from build123d import *

# Parameters (mm, degrees)
ESQUISSE1_R                  = 25
BOSS_EXTRU_1_DEPTH           = 14
ENL_V_START                  = 26
ESQUISSE2_W                  = 9
ESQUISSE2_H                  = 9
ENL_V_MAT_EXTRU_1_DEPTH      = 16
R_P_TITION_CIRCULAIRE1_COUNT = 3
ESQUISSE9_R                  = 11.25
ENL_V_MAT_EXTRU_2_DEPTH      = 16
BOSS_EXTRU_3_START           = -14
BOSS_EXTRU_3_DEPTH           = 20


with BuildPart() as part:
    # Esquisse1 → Boss.-Extru.1 (new body)
    with BuildSketch(Plane.XY):
        Circle(ESQUISSE1_R)
    extrude(amount=BOSS_EXTRU_1_DEPTH)

    # Esquisse2 → Enlèv. mat.-Extru.1 (cut)
    with BuildSketch(Plane(origin=(0, 0, 0), x_dir=(0, 0, -1), z_dir=(1, 0, 0)).offset(ENL_V_START)):
        with Locations((-7, 0)):
            Rectangle(ESQUISSE2_W, ESQUISSE2_H)
    enl_v_mat_extru_1 = extrude(amount=-ENL_V_MAT_EXTRU_1_DEPTH, mode=Mode.SUBTRACT)

    # Répétition circulaire1: Enlèv. mat.-Extru.1 ×3 about axis
    r_p_tition_circulaire1_axis = Axis((0, 0, 0), (0, 0, 1))
    for i in range(1, R_P_TITION_CIRCULAIRE1_COUNT):
        add(enl_v_mat_extru_1.rotate(r_p_tition_circulaire1_axis, i * 360 / R_P_TITION_CIRCULAIRE1_COUNT), mode=Mode.SUBTRACT)

    # Esquisse9 → Enlèv. mat.-Extru.2 (cut)
    with BuildSketch(Plane(origin=(0, 0, 0), x_dir=(-1, 0, 0), z_dir=(0, 0, -1))):
        Circle(ESQUISSE9_R)
    extrude(amount=-ENL_V_MAT_EXTRU_2_DEPTH, mode=Mode.SUBTRACT)

    # Esquisse10 → Boss.-Extru.3 (add)
    with BuildSketch(Plane(origin=(0, 0, 0), x_dir=(-1, 0, 0), z_dir=(0, 0, -1)).offset(BOSS_EXTRU_3_START)):
        Polygon((-15.932437345, 19.265446796), (-21.202216656, 13.246358325), (-17.440286362, 9.952746256), (-12.170507051, 15.971834726), align=None)
    extrude(amount=-BOSS_EXTRU_3_DEPTH)


solid = part.part
Build history of the part. All positions in model axes, mm. A direction names the side the tool comes from. Round coordinates to 2 decimals unless told otherwise and drop trailing zeros. Order: outer loops, then holes, each group sorted by start corner. A loop starts at its lowest first (then second) coordinate and runs counter-clockwise, first axis right, second up. Notation, with made-up numbers: M -32,80.25 L 15,80.25 A21 ccw 15,92.25 Z; hole C -15,-37 d3. An arc over 180 degrees is marked long. Use CSV: the item, a comma, the result in double quotes. Start each with the question number.
(1) Flat gauge pins, fed straight in: P1, Ø6, axis at y = 8.5, z = 22, coming from the -X side; P2, Ø4.5, axis at x = -5.5, y = 13.5, coming from the +Z side; P3, Ø1.5, axis at x = 14.5, z = 8, coming from the +Y side. Where does each tip first touch, or does it go through?
(2) Cut at A-A on x = 0. List the corners of the cut face in (y, z), then the cut area to 3 significant figures.
(3) Mould opens along Y. For faces 1 (the face through (18, 4.5, 7)), 2 (the face through (-12.673, 12.95, 7.063)), 3 (the face through (-12.673, -12.95, 7.063)), 4 (the face through (-4.88, -17.45, 7.06)) say: +Y half, -Y half, draft (parallel to the pull), parting line (faces both ways), or undercut.
(4) Drill centre lines: probe 1 along Z at (x, y) = (15, -2); probe 2 along Y at (x, z) = (0, 10.25); probe 3 along Z at (x, y) = (6, 20.5). Where is each one in solid material? Low to high.
(5) Tool access for faces 5 (the face through (14.84, 12.92, 23.86)), 6 (the face through (-9, -15, 2.5)), 7 (the face through (18.53, 16.3, 23.86)), 8 (the face through (18, 0, 2.5)), 9 (the face through (14.03, 17.6, 23.86)): list every direction of +Z, -Z, +X, -X, +Y, -Y with a clear straight run to the whole face (end or side of a thin tool).
(6) Cut at C-C on y = 18. List the corners of the cut face in (x, z).
(7) Cut at B-B on y = 0. List the corners of the cut face in (x, z).
(8) Cut at D-D on x = 7. List the corners of the cut face in (y, z).
Findings:
1,P1,"stops at x = 16.09"
1,P2,"stops at z = 14"
1,P3,"stops at y = 20.88"
2,outline,"M -25,0 L -11.25,0 L -11.25,14 L -25,14 Z; M 11.25,0 L 25,0 L 25,14 L 11.25,14 Z"
2,area,"385 mm^2"
3,face 1,"undercut"
3,face 2,"+Y half"
3,face 3,"-Y half"
3,face 4,"undercut"
4,probe 1,"z = 0 to 2.5, 11.5 to 14"
4,probe 2,"y = -25 to -11.25, 11.25 to 25"
4,probe 3,"z = 0 to 14"
5,face 5,"+Z, -X, -Y"
5,face 6,"none"
5,face 7,"+Z, +X, +Y"
5,face 8,"+X"
5,face 9,"+Z, -X, +Y"
6,outline,"M -17.35,0 L 17.35,0 L 17.35,14 L 17.04,14 L 17.04,34 L 14.49,34 L 14.49,14 L -17.35,14 Z; hole M -15.59,2.5 L -5.2,2.5 L -5.2,11.5 L -15.59,11.5 Z"
7,outline,"M -25,0 L -11.25,0 L -11.25,14 L -25,14 Z; M 11.25,0 L 25,0 L 25,2.5 L 11.25,2.5 Z; M 11.25,11.5 L 25,11.5 L 25,14 L 11.25,14 Z"
8,outline,"M -24,0 L -8.81,0 L -8.81,14 L -24,14 Z; M 8.81,0 L 24,0 L 24,14 L 8.81,14 Z"
